Autodesk Inventor part; units mm, degrees
ref_plane "YZ Plane" through (0, 0, 0) normal (1, 0, 0) x (0, 1, 0)
ref_plane "XZ Plane" through (0, 0, 0) normal (0, 1, 0) x (-1, 0, 0)
ref_plane "XY Plane" through (0, 0, 0) normal (0, 0, 1) x (1, 0, 0)
sketch "スケッチ1" plane through (0, 0, 0) normal (1, 0, 0) x (0, 1, 0)
  line L0 (0, 0) -> (44, 0)
  line L1 (44, 0) -> (44, -62.8)
  line L2 (44, -62.8) -> (0, -62.8)
  line L3 (0, -62.8) -> (0, 0)
  dimension "d0" = 44
  dimension "d1" = 62.8
extrude "押し出し1" add sketch "スケッチ1" along normal blind 50
sketch "スケッチ2" plane through (50, 0, 0) normal (1, 0, 0) x (0, 0, -1)
  line L0 (0, 44) -> (0, 0)
  line L1 (0, 22) -> (62.8, 22)
  line L2 (62.8, 0) -> (62.8, 44)
  line L3 (62.8, 44) -> (0, 44)
  line L4 (31.4, 44) -> (31.4, 0)
  line L5 (0, 0) -> (62.8, 0)
  line L6 (31.4, 22) -> (51.5, 22)
  line L7 (51.5, 22) -> (51.5, 32.1)
  line L8 (51.5, 32.1) -> (31.4, 32.1)
  line L9 (31.4, 32.1) -> (31.4, 22)
  line L10 (11.3, 22) -> (11.3, 32.1)
  line L11 (11.3, 32.1) -> (31.4, 32.1)
  line L12 (51.5, 22) -> (51.5, 11.9)
  line L13 (51.5, 11.9) -> (31.4, 11.9)
  line L14 (11.3, 11.9) -> (31.4, 11.9)
  line L15 (11.3, 22) -> (11.3, 11.9)
  dimension "d4" = 20.1
  dimension "d5" = 10.1
extrude "押し出し2" cut sketch "スケッチ2" against normal blind 40 contours L10 L11 L4 L1 | L1 L4 L14 L15 | L8 L7 L1 L4 | L1 L12 L13 L4
sketch "スケッチ3" plane through (0, 44, 0) normal (0, 1, 0) x (1, 0, 0)
  line L0 (0, 0) -> (50, 0)
  line L1 (10, 0) -> (10, 62.8)
  line L2 (0, 62.8) -> (50, 62.8)
  line L3 (0, 62.8) -> (0, 0)
  line L4 (0, 31.4) -> (50, 31.4)
  line L5 (50, 0) -> (50, 62.8)
  line L6 (10, 41.4) -> (50, 41.4)
  point P0 (20, 41.4)
  point P1 (40, 41.4)
  point P2 (20, 21.4)
  point P3 (40, 21.4)
  dimension "d8" = 10
  dimension "d9" = 10
  dimension "d10" = 10
  dimension "d11" = 20
hole "穴1" at (20, 44, -41.4) at (40, 44, -41.4) at (20, 44, -21.4) at (40, 44, -21.4) direction (0, -1, 0) diameter 3.3 end through all
fillet "フィレット1" radius 5 4 edges at (25, 44, 0) (25, 0, 0) (25, 0, -62.8) (25, 44, -62.8)
sketch "スケッチ4" plane through (10, 0, 0) normal (1, 0, 0) x (0, 0, -1)
  line L0 (11.3, 11.9) -> (11.3, 32.1)
  line L1 (11.3, 22) -> (51.5, 22)
  line L2 (51.5, 32.1) -> (51.5, 11.9)
  line L3 (11.3, 32.1) -> (51.5, 32.1)
  line L4 (31.4, 32.1) -> (31.4, 11.9)
  line L5 (51.5, 11.9) -> (11.3, 11.9)
  point P0 (0, 0)
  point P1 (41.4, 22)
  point P2 (21.4, 22)
  dimension "d20" = 10
hole "穴2" at (10, 22, -41.4) at (10, 22, -21.4) direction (-1, 0, 0) diameter 3.3 end through all
fillet "フィレット2" radius 1 4 edges at (50, 22, -51.5) (50, 11.9, -31.4) (50, 32.1, -31.4) (50, 22, -11.3)
sketch "スケッチ5" plane through (50, 0, 0) normal (1, 0, 0) x (0, 0, -1)
  line L0 (57.8, 44) -> (5, 44)
  line L1 (31.4, 44) -> (31.4, 33.1)
  line L2 (52.5, 33.1) -> (10.3, 33.1)
  line L3 (31.4, 44) -> (36.4, 44)
  line L4 (36.4, 44) -> (36.4, 34)
  line L5 (36.4, 34) -> (31.4, 34)
  line L6 (31.4, 34) -> (31.4, 44)
  line L7 (26.4, 44) -> (26.4, 34)
  line L8 (26.4, 34) -> (31.4, 34)
  point P0 (0, 0)
  point P1 (26.4, 44)
  dimension "d29" = 10
  dimension "d30" = 5
extrude "押し出し3" cut sketch "スケッチ5" against normal blind 100
properties part number "framefixpart1_forearm"
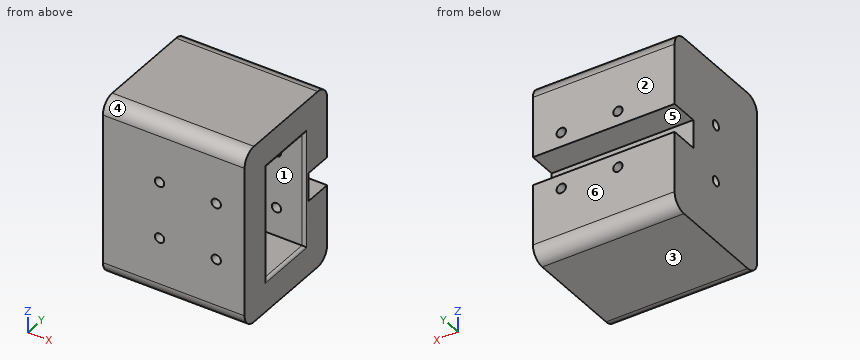
CAD build for the part. Positions are in the model's coordinates, mm. Face numbers are marked on the shaded views. A direction names the side the tool comes from. Coordinates: 2 decimals unless noted, no trailing zeros. Order: outer loops, then holes, each group sorted by start corner. A loop starts at its lowest first (then second) coordinate and runs counter-clockwise, first axis right, second up. Notation, with made-up numbers: M 25.5,61 L 62.5,61 A28 cw 62.5,84 Z; hole C 1,-25.5 d1. An arc over 180 degrees is marked long. Write each question's results on one line, items separated by ' | '. Start each with the question number.
Q1. Flat gauge pins, fed straight in: P1, Ø8, axis at x = 43, y = 19, coming from the +Z side; P2, Ø3, axis at x = 13, z = -30.5, coming from the +Y side. Where does each tip first touch, or does it go through?
Q2. Which spindle directions (+Z, -Z, +X, -X, +Y, -Y) get a long thin tool onto all of the face, cutting with end or side? Do the marked faces 1 and 2. Say none if no direction does.
Q3. Pull direction Z, two halves, no side cores. Call the marked faces 3, 4, 5 and 6: +Z half, -Z half, draft (parallel to the pull), parting line (faces both ways), or undercut.
Q4. Drill centre lines: probe 1 along X at (y, z) = (3, -41.4); probe 2 along Z at (x, y) = (20, 37); probe 3 along Z at (x, y) = (5.75, 22). Where is each one in solid material? Low to high. Write a range as from..to.
Q5. Cut at B-B (y = 22). List the corners of the cut face in (x, z), then the cut area to 3 significant figures.
Q6. Cut at D-D (x = 25). List the corners of the cut face in (y, z).
Q7. Cut at A-A (x = 40). Count the separate pieces of the cut face and the enclosed holes in it, then the cut area to 3 significant figures.
Found:
1) P1: z = 0 | P2: y = 34
2) face 1: +X | face 2: +Z, -Z, +X, -X, +Y
3) face 3: -Z half | face 4: +Z half | face 5: undercut | face 6: draft
4) probe 1: 0..18.35, 21.65..38.35, 41.65..50 | probe 2: -62.8..-43.05, -39.75..-36.4, -26.4..-23.05, -19.75..0 | probe 3: -62.8..-43.05, -39.75..-23.05, -19.75..0
5) outline: M 0,-62.8 L 50,-62.8 L 50,-52.5 A1 ccw 49,-51.5 L 10,-51.5 L 10,-43.05 L 0,-43.05 Z; M 0,-39.75 L 10,-39.75 L 10,-23.05 L 0,-23.05 Z; M 0,-19.75 L 10,-19.75 L 10,-11.3 L 49,-11.3 A1 ccw 50,-10.3 L 50,0 L 0,0 Z | area: 1,470 mm²
6) outline: M 0,-57.8 A5 ccw 5,-62.8 L 39,-62.8 A5 ccw 44,-57.8 L 44,-36.4 L 34,-36.4 L 34,-26.4 L 44,-26.4 L 44,-5 A5 ccw 39,0 L 5,0 A5 ccw 0,-5 Z; hole M 11.9,-51.5 L 32.1,-51.5 L 32.1,-11.3 L 11.9,-11.3 Z
7) separate pieces: 4 | enclosed holes: 0 | area: 1,670 mm²
